Verification items for this drawing (mm, ordinates from the low corner). Give positions to 0.01 mm unless a question says otherwise; leave off trailing zeros. Order: outer loops, then holes, each group sorted by start corner. A loop starts at its lowest first (then second) coordinate and runs counter-clockwise, first axis right, second up. Notation, with made-up numbers: (18, 67) -> (64, 67) arc R24 cw to (64, 102) -> close; hole circle Ø2 at (-1.75, 51). An arc over 180 degrees is marked (long way). One line per question, with ' | ' between items.
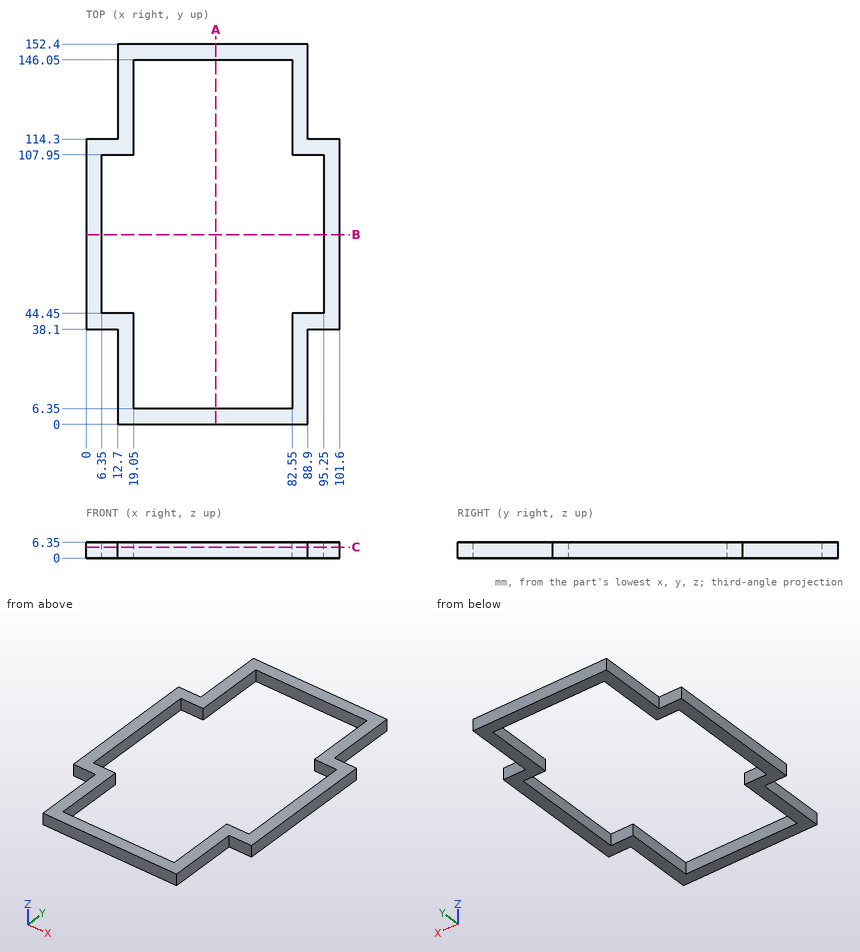
Q1. Depth check by flat-ended pin: pin 1 Ø1.9 at (y, z) = (24.5, 3) entering from -X; pin 2 Ø1.9 at (x, z) = (4.5, 3) entering from -Y. Enter the tip coordinate at first touch or a pass-through.
Result sheet:
pin 1: stops at x = 12.7 | pin 2: stops at y = 38.1
Q2. Thickness scan on line 1 (X direction, y = 45, z = 6); line 2 (Y direction, x = 24.5, z = 0.75); line 3 (X direction, y = 137.5, z = 2). Record the ranges inside material, lowest first.
Result sheet:
line 1: x = 0 to 6.35, 95.25 to 101.6 | line 2: y = 0 to 6.35, 146.05 to 152.4 | line 3: x = 12.7 to 19.05, 82.55 to 88.9
Q3. Section check C-C (z = 4.5). Enter the section's corners in (x, y), and give its area (3 significant figures).
Result sheet:
outline: (0, 38.1) -> (12.7, 38.1) -> (12.7, 0) -> (88.9, 0) -> (88.9, 38.1) -> (101.6, 38.1) -> (101.6, 114.3) -> (88.9, 114.3) -> (88.9, 152.4) -> (12.7, 152.4) -> (12.7, 114.3) -> (0, 114.3) -> close; hole (6.35, 44.45) -> (19.05, 44.45) -> (19.05, 6.35) -> (82.55, 6.35) -> (82.55, 44.45) -> (95.25, 44.45) -> (95.25, 107.95) -> (82.55, 107.95) -> (82.55, 146.05) -> (19.05, 146.05) -> (19.05, 107.95) -> (6.35, 107.95) -> close | area: 3,060 mm2
Q4. Section check B-B (y = 76). Enter the section's corners in (x, z), and give its area (3 significant figures).
Result sheet:
outline: (0, 0) -> (6.35, 0) -> (6.35, 6.35) -> (0, 6.35) -> close; (95.25, 0) -> (101.6, 0) -> (101.6, 6.35) -> (95.25, 6.35) -> close | area: 80.6 mm2
Q5. Section check A-A (x = 52). Enter the section's corners in (y, z), and give its area (3 significant figures).
Result sheet:
outline: (0, 0) -> (6.35, 0) -> (6.35, 6.35) -> (0, 6.35) -> close; (146.05, 0) -> (152.4, 0) -> (152.4, 6.35) -> (146.05, 6.35) -> close | area: 80.6 mm2
